```python
from build123d import *

# Parameters (mm, degrees)
CUT_EXTRUDE1_START = 1.397
CUT_EXTRUDE1_DEPTH = 10.7188
CIRPATTERN1_COUNT  = 21
SKETCH4_R          = 1.5875
CUT_EXTRUDE2_DEPTH = 31.241836167
CUT_EXTRUDE3_DEPTH = 1.190625
CIRPATTERN2_COUNT  = 2
CIRPATTERN2_ANGLE  = 90
CUT_EXTRUDE4_DEPTH = 50.8
SKETCH8_R          = 12.7
CUT_EXTRUDE5_DEPTH = 50.8


with BuildPart() as part:
    # Sketch2 → Revolve1 (revolve)
    with BuildSketch(Plane(origin=(0, 0, 0), x_dir=(0, 0, -1), z_dir=(1, 0, 0)), mode=Mode.PRIVATE) as revolve1_sk:
        with BuildLine():
            Line((-11.1125, 3.175), (11.1125, 3.175))
            Line((11.1125, 3.175), (11.1125, 19.8882))
            Line((11.1125, 19.8882), (10.21715, 19.8882))
            ThreePointArc((10.21715, 19.8882), (9.559562343, 19.158250378), (9.3218, 18.204983865))
            Line((9.3218, 18.204983865), (9.3218, 16.521767729))
            Line((9.3218, 16.521767729), (-1.397, 16.521767729))
            Line((-1.397, 16.521767729), (-1.397, 18.204983865))
            ThreePointArc((-1.397, 18.204983865), (-1.634762343, 19.158250378), (-2.29235, 19.8882))
            Line((-2.29235, 19.8882), (-3.1877, 19.8882))
            Line((-3.1877, 19.8882), (-3.1877, 11.9126))
            Line((-3.1877, 11.9126), (-11.1125, 11.9126))
            Line((-11.1125, 11.9126), (-11.1125, 3.175))
        make_face()
    revolve(revolve1_sk.sketch.rotate(Axis((0, 0, 11.1125), (0, 0, -1)), 90), axis=Axis((0, 0, 11.1125), (0, 0, -1)))

    # Sketch3 → Cut-Extrude1 (cut)
    with BuildSketch(Plane.XY.offset(CUT_EXTRUDE1_START)):
        with BuildLine():
            Line((-0.690489274, 15.2019), (0.690489274, 15.2019))
            Line((0.690489274, 15.2019), (1.2827, 16.4719))
            ThreePointArc((1.2827, 16.4719), (0, 16.521767729), (-1.2827, 16.4719))
            Line((-1.2827, 16.4719), (-0.690489274, 15.2019))
        make_face()
    cut_extrude1 = extrude(amount=-CUT_EXTRUDE1_DEPTH, mode=Mode.SUBTRACT)

    # CirPattern1: Cut-Extrude1 ×21 about axis
    cirpattern1_axis = Axis((0, 0, 0), (0, 0, 1))
    for i in range(1, CIRPATTERN1_COUNT):
        add(cut_extrude1.rotate(cirpattern1_axis, i * 360 / CIRPATTERN1_COUNT), mode=Mode.SUBTRACT)

    # Sketch4 → Cut-Extrude2 (cut, through all)
    with BuildSketch(Plane(origin=(0, 0, 0), x_dir=(1, 0, 0), z_dir=(0, 1, 0))):
        with Locations(Location((0, -7.1501, 0), (0, 0, 90))):
            Circle(SKETCH4_R)
    cut_extrude2 = extrude(amount=CUT_EXTRUDE2_DEPTH, mode=Mode.SUBTRACT)

    # Sketch5 → Revolve2 (revolve)
    with BuildSketch(Plane.XY.offset(7.1501), mode=Mode.PRIVATE) as revolve2_sk:
        Polygon((1.0795, 11.806349246), (1.5875, 11.298349246), (1.5875, 3.81), (0.9525, 3.175), (0, 3.175), (0, 11.806349246), align=None)
    revolve2 = revolve(revolve2_sk.sketch.rotate(Axis((0, 0, 7.1501), (0, 1, 0)), 90), axis=Axis((0, 0, 7.1501), (0, 1, 0)))

    # Sketch6 → Cut-Extrude3 (cut)
    with BuildSketch(Plane(origin=(0, 11.806349246, 0), x_dir=(1, 0, 0), z_dir=(0, 1, 0))):
        Polygon((0, -6.233556448), (-0.79375, -6.691828224), (-0.79375, -7.608371776), (0, -8.066643552), (0.79375, -7.608371776), (0.79375, -6.691828224), align=None)
    cut_extrude3 = extrude(amount=-CUT_EXTRUDE3_DEPTH, mode=Mode.SUBTRACT)

    # CirPattern2: Cut-Extrude2, Revolve2, Cut-Extrude3 ×2 about axis
    cirpattern2_axis = Axis((0, 0, 0), (0, 0, -1))
    add([cut_extrude2.rotate(cirpattern2_axis, i * CIRPATTERN2_ANGLE / (CIRPATTERN2_COUNT - 1)) for i in range(1, CIRPATTERN2_COUNT)], mode=Mode.SUBTRACT)
    add([revolve2.rotate(cirpattern2_axis, i * CIRPATTERN2_ANGLE / (CIRPATTERN2_COUNT - 1)) for i in range(1, CIRPATTERN2_COUNT)])
    add([cut_extrude3.rotate(cirpattern2_axis, i * CIRPATTERN2_ANGLE / (CIRPATTERN2_COUNT - 1)) for i in range(1, CIRPATTERN2_COUNT)], mode=Mode.SUBTRACT)

    # Sketch7 → Cut-Extrude4 (cut)
    with BuildSketch(Plane.XY.offset(11.1125)):
        Polygon((0, 3.886144662), (-3.3655, 1.943072331), (-3.3655, -1.943072331), (0, -3.886144662), (3.3655, -1.943072331), (3.3655, 1.943072331), align=None)
    extrude(amount=-CUT_EXTRUDE4_DEPTH, mode=Mode.SUBTRACT)

    # Sketch8 → Cut-Extrude5 (cut)
    with BuildSketch(Plane.XY.offset(3.1877)):
        Circle(SKETCH8_R)
    extrude(amount=CUT_EXTRUDE5_DEPTH, mode=Mode.SUBTRACT)


solid = part.part
```
Geometry: final body of the model. Coordinates: model frame, mm. A direction names the side the tool comes from. Coordinates: 2 decimals unless noted, no trailing zeros. Answer as CSV lines item,"result".
Q1. Line query: probe 1 along Y at (x, z) = (13, -9); probe 2 along Z at (x, y) = (-11, 14); probe 3 along X at (y, z) = (7, -1.5). Output: solid intervals per line, ascending. Write a range as [from, to].
Answers:
probe 1,"y = [-10.2, -8.46], [-7.89, 9.1]"
probe 2,"z = [-11.11, -9.32], [1.4, 3.19]"
probe 3,"x = [-14.66, 14.66]"
Q2. Draft query along Y for faces 5 (the flat face through (-3.331, -15.505, -3.887)), 6 (the flat face through (15.21, -4.48, -3.89)), 7 (the cylindrical face through (7.154, 14.893, -3.887)). Return one class per face: pulls with the +Y half, pulls with the -Y half, needs draft (parallel to the pull), parting line crosses it, or undercut.
Answers:
face 5,"pulls with the -Y half"
face 6,"undercut"
face 7,"pulls with the +Y half"
Q3. Set-up query: faces 1 (the flat face through (-11.486, -10.935, -3.887)), 2 (the flat face through (14.823, -3.373, -3.887)), 3 (the flat face through (4.47, 14.53, -3.89)), 4 (the cylindrical face through (14.3, 8.275, -3.887)). Return all of +Z, -Z, +X, -X, +Y, -Y with unobstructed straight access to the full face (end or side cutting, diameter ignored); none if empty.
Answers:
face 1,"-Y"
face 2,"+X"
face 3,"+Y"
face 4,"+X, +Y"
Q4. First-contact query: P1, Ø1.5, axis at x = 0, z = -4, coming from the +Y side; P2, Ø6, axis at x = 14.5, z = -2, coming from the -Y side; P3, Ø5, axis at y = 6, z = -3.5, coming from the -X side. Flat tips, straight axial feed; report the tip coordinate or a pass-through.
Answers:
P1,"stops at y = 15.33"
P2,"stops at y = -11.2"
P3,"stops at x = -16.15"
